```python
from build123d import *

# Parameters (mm, degrees)
SKETCH1_W           = 250
SKETCH1_H           = 150
BOSS_EXTRUDE1_DEPTH = 150


with BuildPart() as part:
    # Sketch1 → Boss-Extrude1 (new body)
    with BuildSketch(Plane.XY):
        with Locations((0, 75)):
            Rectangle(SKETCH1_W, SKETCH1_H)
    boss_extrude1 = extrude(amount=-BOSS_EXTRUDE1_DEPTH)

    # Sketch2 → Cut-Revolve1 (revolve, cut)
    with BuildSketch(Plane.XY):
        Polygon((0, 150), (87, 150), (87, 123), (85, 121), (74, 121), (72, 119), (72, 96), (70, 94), (61, 94), (59, 92), (59, 46), (57, 44), (43, 44), (41, 42), (41, 36), (39, 34), (0, 34), align=None)
    cut_revolve1 = revolve(axis=Axis((0, 0, 0), (0, 1, 0)), mode=Mode.SUBTRACT)

    # Mirror1: Boss-Extrude1, Cut-Revolve1 across plane
    add(boss_extrude1.mirror(Plane(origin=(0, 0, 0), x_dir=(1, 0, 0), z_dir=(0, 0, -1))))
    add(cut_revolve1.mirror(Plane(origin=(0, 0, 0), x_dir=(1, 0, 0), z_dir=(0, 0, -1))), mode=Mode.SUBTRACT)


solid = part.part
```
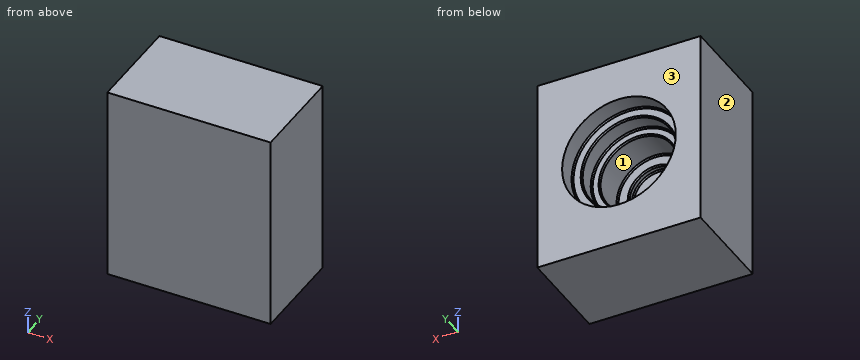
CAD build for the part. Positions are in the model's coordinates, mm. Face numbers are marked on the shaded views. Coordinates: 2 decimals unless noted, no trailing zeros. Write each loop counter-clockwise with the first axis right and the second up, starting at its lowest first coordinate (ties: lowest second). Pieces come first, ordered by that corner, then holes.
(1) Drill centre lines: probe 1 along Z at (x, y) = (0, 59); probe 2 along Z at (x, y) = (0, 105.75); probe 3 along Y at (x, z) = (-17, 51). Where is each one in solid material? Low to high.
(2) Cut at D-D, the plane y = 51.5. List the corners of the cut face in (x, z), and give its area (3 significant figures).
(3) Cut at A-A, the plane y = 134.5. List the corners of the cut face in (x, z), and give its area (3 significant figures).
(4) Two-plate mould, pull along X, no slides. Class the marked faces 1, 2 and 3: +X half, -X half, draft (parallel to the pull), parting line (faces both ways), or undercut.
Geometry says:
1. probe 1: z = -150 to -59, 59 to 150
1. probe 2: z = -150 to -72, 72 to 150
1. probe 3: y = 0 to 44
2. outline: (-125, -150) - (125, -150) - (125, 150) - (-125, 150) - close; hole circle Ø118 at (0, 0)
2. area: 64,100 mm2
3. outline: (-125, -150) - (125, -150) - (125, 150) - (-125, 150) - close; hole circle Ø174 at (0, 0)
3. area: 51,200 mm2
4. face 1: undercut
4. face 2: -X half
4. face 3: draft
